Build history of the part. All positions in model axes, mm. A direction names the side the tool comes from. Give positions to 0.01 mm unless a question says otherwise; leave off trailing zeros. Loops run counter-clockwise (first coordinate to the right, second up) from the corner with the lowest first, then second, coordinate; pieces in that order, holes last.
1) Band-saw the part on C-C on x = 0. List the corners of the cut face in (y, z), then the cut area to 3 significant figures.
2) Two-plate mould, pull along X, no slides. Class faces 4 (the flat face through (1, 0, -2)), 5 (the flat face through (32, 18, -36)), 6 (the flat face through (38, 10, -19)), 7 (the flat face through (-32, 18, -36)): +X half, -X half, draft (parallel to the pull), parting line (faces both ways), or undercut.
3) Band-saw the part on A-A on y = 21.5. List the corners of the cut face in (x, z).
4) Wall check: line 1 (X direction, y = 23, z = -46); line 2 (Z direction, x = -35, y = 21.25); line 3 (X direction, y = 10.5, z = -31). Give the ranges that are in metal, low to high.
5) 3-axis set-ups, long thin cutter, end or side, ignore diameter. For faces 1 (the flat face through (41, 5, 92)), 2 (the flat face through (-35, 18, -56)), 3 (the flat face through (-35, 18, -16)): which of +Z, -Z, +X, -X, +Y, -Y reach the whole face in a straight line?
6) Band-saw the part on B-B on z = 65. List the corners of the cut face in (x, y).
7) Flat gauge pins, fed straight in: P1, Ø5, axis at x = 34, y = 18.5, coming from the +Z side; P2, Ø13, axis at y = 20.5, z = -43, coming from the -X side; P3, Ø10, axis at y = 8, z = 22, coming from the +X side; P4, Ø3.5, axis at x = 35, z = -26, coming from the -Y side. Where does each tip first touch, or does it go through?
```python
from build123d import *

# Parameters (mm, degrees)
EXTRUDE_1_DEPTH     = 10
SKETCH_4_W          = 6
SKETCH_4_H          = 40
EXTRUDE_3_DEPTH     = 16
SKETCH_7_R          = 1.5
CUT_EXTRUDE_3_DEPTH = 10
EXTRUDE_4_DEPTH     = 10


with BuildPart() as part:
    # 草图1 → 凸台-拉伸1 (new body)
    with BuildSketch(Plane(origin=(0, 0, 0), x_dir=(1, 0, 0), z_dir=(0, 1, 0))):
        with BuildLine():
            Line((-38, -75), (-38, 75))
            ThreePointArc((-38, 75), (0, 113), (38, 75))
            Line((38, 75), (38, -75))
            ThreePointArc((38, -75), (0, -113), (-38, -75))
        make_face()
    extrude(amount=EXTRUDE_1_DEPTH)

    # 草图4 → 凸台-拉伸3 (add)
    with BuildSketch(Plane(origin=(0, 10, 0), x_dir=(1, 0, 0), z_dir=(0, 1, 0))):
        with Locations((-35, 36)):
            Rectangle(SKETCH_4_W, SKETCH_4_H)
        with Locations((35, 36)):
            Rectangle(SKETCH_4_W, SKETCH_4_H)
    extrude(amount=EXTRUDE_3_DEPTH)

    # 草图7 → 切除-拉伸3 (cut)
    with BuildSketch(Plane(origin=(0, 26, 0), x_dir=(1, 0, 0), z_dir=(0, 1, 0))):
        with Locations((-35, 26)):
            Circle(SKETCH_7_R)
        with Locations((-35, 46)):
            Circle(SKETCH_7_R)
        with Locations((35, 26)):
            Circle(SKETCH_7_R)
        with Locations((35, 46)):
            Circle(SKETCH_7_R)
    extrude(amount=-CUT_EXTRUDE_3_DEPTH, mode=Mode.SUBTRACT)

    # 草图8 → 凸台-拉伸4 (add)
    with BuildSketch(Plane(origin=(0, 10, 0), x_dir=(1, 0, 0), z_dir=(0, 1, 0))):
        with BuildLine():
            Line((-47, -72), (47, -72))
            ThreePointArc((47, -72), (52.310885546, -73.526836794), (56, -77.641101056))
            Line((56, -77.641101056), (56, -86.358898944))
            ThreePointArc((56, -86.358898944), (52.310885546, -90.473163206), (47, -92))
            Line((47, -92), (-47, -92))
            ThreePointArc((-47, -92), (-52.310885546, -90.473163206), (-56, -86.358898944))
            Line((-56, -86.358898944), (-56, -77.641101056))
            ThreePointArc((-56, -77.641101056), (-52.310885546, -73.526836794), (-47, -72))
        make_face()
    extrude(amount=-EXTRUDE_4_DEPTH)


solid = part.part
```
Findings below:
1. outline: (0, -113) - (10, -113) - (10, 113) - (0, 113) - close
1. area: 2,260 mm2
2. face 4: draft
2. face 5: undercut
2. face 6: +X half
2. face 7: undercut
3. outline: (-38, -56) - (-32, -56) - (-32, -16) - (-38, -16) - close; (32, -56) - (38, -56) - (38, -16) - (32, -16) - close; hole circle Ø3 at (-35, -46); hole circle Ø3 at (-35, -26); hole circle Ø3 at (35, -46); hole circle Ø3 at (35, -26)
4. line 1: x = -38 to -36.5, -33.5 to -32, 32 to 33.5, 36.5 to 38
4. line 2: z = -56 to -47.5, -44.5 to -27.5, -24.5 to -16
4. line 3: x = -38 to -32, 32 to 38
5. face 1: +Z, +X, +Y, -Y
5. face 2: -Z, +X, -X, +Y
5. face 3: +Z, +X, -X, +Y
6. outline: (-38, 0) - (38, 0) - (38, 10) - (-38, 10) - close
7. P1: stops at z = -16
7. P2: stops at x = -38
7. P3: stops at x = 38
7. P4: stops at y = 0
